Check sheet for the modelled part. Datum: model origin and axes. Units: mm. A direction names the side the tool comes from. Round coordinates to 2 decimals unless told otherwise and drop trailing zeros. Loops run counter-clockwise (first coordinate to the right, second up) from the corner with the lowest first, then second, coordinate; pieces in that order, holes last. Notation, with made-up numbers: (50, 47.25) -> (106, 47.25) arc R15 ccw to (106, 71.25) -> close; hole circle Ø10 at (61.25, -23.75). An arc over 180 degrees is marked (long way). Use one line per item in the form item = value. Start each with the question number.
(1) Sectioned sample at B-B (y = 2). Record the cut outline in (x, z).
(2) Set-up check for faces 1 (the cylindrical face through (8.5, 5.5, 0)), 2 (the cylindrical face through (-8.5, 5.5, 0)), 3 (the cylindrical face through (2, 5.5, 9.8)), 4 (the cylindrical face through (-4.57, 1.479, -7.167)): record each of +Z, -Z, +X, -X, +Y, -Y from which the full face is reachable in a straight line by a thin tool's end or side.
(3) Sectioned sample at D-D (x = 6.75). Record the cut outline in (y, z).
(4) Sectioned sample at C-C (z = 7). Record the cut outline in (x, y).
(5) Draft check along X on faces 5 (the flat face through (4, 12, 0)), 6 (the cylindrical face through (1.88, 7.56, -2.95)), 7 (the cylindrical face through (3.8, 9.97, -2.41)). Enter one of: released by +X, released by -X, zero draft, split by the parting line, or undercut.
(6) Sectioned sample at A-A (x = -2.75). Record the cut outline in (y, z).
(7) Material ranges on probe 1 along X at (y, z) = (7.5, 0); probe 2 along Z at (x, y) = (0, 2.15); probe 3 along X at (y, z) = (9, 0), recorded low to high. Write a range as [from, to].
(8) Go/stop test with flat-tipped pins: pin 1 (11 mm diameter, centred on x = 0, z = 0, fed in from -Y); pin 2 (5 mm diameter, centred on x = -6.5, y = 4.5, fed in from +Z); pin 3 (1.5 mm diameter, centred on x = -5, z = -7.5, fed in from +Y). Record where each tip stops, or that it passes through.
Autodesk Inventor part; units mm, degrees
ref_plane "YZ Plane" through (0, 0, 0) normal (1, 0, 0) x (0, 1, 0)
ref_plane "XZ Plane" through (0, 0, 0) normal (0, 1, 0) x (-1, 0, 0)
ref_plane "XY Plane" through (0, 0, 0) normal (0, 0, 1) x (1, 0, 0)
sketch "Эскиз1" plane through (0, 0, 0) normal (0, 1, 0) x (-1, 0, 0)
  circle A0 centre (0, 0) radius 11.5
  circle A1 centre (0, 0) radius 8.5
  dimension "d0" = 23
  dimension "d1" = 17
extrude "Выдавливание1" add sketch "Эскиз1" along normal blind 3
sketch "Эскиз2" plane through (0, 3, 0) normal (0, 1, 0) x (1, 0, 0)
  circle A0 centre (0, 0) radius 10
  circle A1 centre (-10, 0) radius 1.5
  circle A2 centre (-9.2388, -3.8268) radius 1.5
  circle A3 centre (-7.0711, -7.0711) radius 1.5
  circle A4 centre (-3.8268, -9.2388) radius 1.5
  circle A5 centre (0, -10) radius 1.5
  circle A6 centre (3.8268, -9.2388) radius 1.5
  circle A7 centre (7.0711, -7.0711) radius 1.5
  circle A8 centre (9.2388, -3.8268) radius 1.5
  circle A9 centre (10, 0) radius 1.5
  circle A10 centre (9.2388, 3.8268) radius 1.5
  circle A11 centre (7.0711, 7.0711) radius 1.5
  circle A12 centre (3.8268, 9.2388) radius 1.5
  circle A13 centre (0, 10) radius 1.5
  circle A14 centre (-3.8268, 9.2388) radius 1.5
  circle A15 centre (-7.0711, 7.0711) radius 1.5
  circle A16 centre (-9.2388, 3.8268) radius 1.5
  point P0 (-8.5625, 5.1657)
  point P1 (-9.7073, 2.4019)
  point P2 (-9.8875, 1.4958)
  point P3 (-9.8875, -1.4958)
  point P4 (-9.7073, -2.4019)
  point P5 (-8.5625, -5.1657)
  point P6 (-8.0492, -5.9338)
  point P7 (-5.9338, -8.0492)
  point P8 (-5.1657, -8.5625)
  point P9 (-2.4019, -9.7073)
  point P10 (-1.4958, -9.8875)
  point P11 (1.4958, -9.8875)
  point P12 (2.4019, -9.7073)
  point P13 (5.1657, -8.5625)
  point P14 (5.9338, -8.0492)
  point P15 (8.0492, -5.9338)
  point P16 (8.5625, -5.1657)
  point P17 (9.7073, -2.4019)
  point P18 (9.8875, -1.4958)
  point P19 (9.8875, 1.4958)
  point P20 (9.7073, 2.4019)
  point P21 (8.5625, 5.1657)
  point P22 (8.0492, 5.9338)
  point P23 (5.9338, 8.0492)
  point P24 (5.1657, 8.5625)
  point P25 (2.4019, 9.7073)
  point P26 (1.4958, 9.8875)
  point P27 (-1.4958, 9.8875)
  point P28 (-2.4019, 9.7073)
  point P29 (-5.1657, 8.5625)
  point P30 (-5.9338, 8.0492)
  point P31 (-8.0492, 5.9338)
  dimension "d4" = 20
  dimension "d5" = 3
  dimension "d8" = 360
extrude "Выдавливание2" add sketch "Эскиз2" along normal blind 5 contours A9 A0 A8 A7 A6 A5 A4 A3 A2 A1 A16 A15 A14 A13 A12 A11 A10
sketch "Эскиз3" plane through (0, 8, 0) normal (0, 1, 0) x (1, 0, 0)
  circle A0 centre (0, 0) radius 4.5
  circle A1 centre (0, 0) radius 3.5
  dimension "d12" = 9
  dimension "d13" = 7
extrude "Выдавливание3" add sketch "Эскиз3" along normal blind 4
sketch "Эскиз4" plane through (0, 8, 0) normal (0, 1, 0) x (1, 0, 0)
  circle A0 centre (0, 0) radius 3.5
extrude "Выдавливание4" cut sketch "Эскиз4" against normal through all
sketch "Эскиз5" plane through (0, 3, 0) normal (0, -1, 0) x (1, 0, 0)
  circle A0 centre (0, 0) radius 3.5
  circle A1 centre (0, 0) radius 3.5
  circle A2 centre (0, 3.5) radius 1
  circle A3 centre (-3.0311, -1.75) radius 1
  circle A4 centre (3.0311, -1.75) radius 1
  point P0 (-0.9897, 3.3571)
  point P1 (0.9897, 3.3571)
  point P2 (3.4022, -0.8214)
  point P3 (2.4125, -2.5357)
  point P4 (-3.4022, -0.8214)
  point P5 (-2.4125, -2.5357)
  dimension "d18" = 2
  dimension "d21" = 360
extrude "Выдавливание5" add sketch "Эскиз5" against normal blind 6 contours A2 A0 | A0 A4 | A3 A0 picked at (0, 3.156) picked at (2.7332, -1.578) picked at (-2.7274, -1.5885)
sketch "Эскиз6" plane through (0, 12, 0) normal (0, 1, 0) x (1, 0, 0)
  arc A0 (2.4125, 2.5357) -> (3.4022, 0.8214) centre (3.0311, 1.75) ccw
  line L0 (0, 0) -> (3.0311, 1.75)
  line L1 (0, 0) -> (-4.9072, -2.8332)
  line L2 (-4.6871, -3.8608) -> (-2.1071, -2.3712)
  line L3 (-2.1071, -2.3712) -> (-3.1071, -0.6392)
  line L4 (-3.1071, -0.6392) -> (-5.6871, -2.1288)
  line L5 (-5.6871, -2.1288) -> (-4.6871, -3.8608)
  circle A1 centre (0, 0) radius 4.5
  line L6 (-4.6871, -3.8608) -> (-3.1071, -0.6392) construction
  line L7 (-2.1071, -2.3712) -> (-5.6871, -2.1288) construction
  point P0 (-3.8971, -2.25)
  dimension "d25" = 2
extrude "Выдавливание6" cut sketch "Эскиз6" against normal blind 4 contours L3 L2 A1 L1 | L1 A1 L4 L3 | A1 L2 L5 L4
properties part number "вращалка"
Checks:
q1.outline = circle Ø23 at (0, 0); hole circle Ø17 at (0, 0)
q2.face_1 = +X, +Y
q2.face_2 = -X, +Y
q2.face_3 = +Z, +X, +Y
q2.face_4 = -Y
q3.outline = (0, -9.31) -> (3, -9.31) -> (3, -5.61) -> (8, -5.61) -> (8, 5.61) -> (3, 5.61) -> (3, 9.31) -> (0, 9.31) -> (0, 5.17) -> (3, 5.17) -> (3, -5.17) -> (0, -5.17) -> close
q4.outline = (-9.12, 0) -> (-4.82, 0) -> (-4.82, 3) -> (4.82, 3) -> (4.82, 0) -> (9.12, 0) -> (9.12, 3) -> (5.57, 3) -> (5.57, 8) -> (-5.57, 8) -> (-5.57, 3) -> (-9.12, 3) -> close
q5.face_5 = zero draft
q5.face_6 = undercut
q5.face_7 = split by the parting line
q6.outline = (0, -11.17) -> (3, -11.17) -> (3, -8.19) -> (8, -8.19) -> (8, -3.56) -> (12, -3.56) -> (12, -2.17) -> (9, -2.17) -> (9, -0.79) -> (3, -0.79) -> (3, -8.04) -> (0, -8.04) -> close; (0, 8.04) -> (3, 8.04) -> (3, 2.17) -> (8, 2.17) -> (8, 2.74) -> (12, 2.74) -> (12, 3.56) -> (8, 3.56) -> (8, 8.19) -> (3, 8.19) -> (3, 11.17) -> (0, 11.17) -> close
q7.probe_1 = [-8.5, -3.5], [3.5, 8.5]
q7.probe_2 = [-11.5, -8.5], [8.5, 11.5]
q7.probe_3 = [-4.5, -3.5], [3.5, 4.5]
q8.pin_1 = 3
q8.pin_2 = 10.58
q8.pin_3 = 8
